Solid Edge part; units mm, degrees
sketch "Sketch1" plane through (0, 0, 0) normal (0, 0, 1) x (1, 0, 0)
  line L0 (20, -15) -> (-20, -15)
  line L1 (-20, -15) -> (-20, 15)
  line L2 (-20, 15) -> (20, 15)
  line L3 (20, 15) -> (20, -15)
extrude "Protrusion1" add sketch "Sketch1" along normal blind 2
sketch "Sketch2" plane through (0, 0, 0) normal (0, 0, -1) x (1, 0, 0)
  line L0 (6.25, -11.5) -> (6.25, 11.5)
  line L1 (6.25, 11.5) -> (-6.25, 11.5)
  line L2 (-6.25, 11.5) -> (-6.25, -11.5)
  line L3 (-6.25, -11.5) -> (6.25, -11.5)
extrude "ExtrudedProtrusion_2" add sketch "Sketch2" along normal blind 6
sketch "Sketch3" plane through (-20, 0, 1) normal (-1, 0, 0) x (0, -1, 0)
  line L0 (-15, 17.5) -> (-15, 1)
  line L1 (-15, 1) -> (15, 1)
  line L2 (15, 1) -> (15, 2.5)
  arc A0 (17, 4.5) -> (15, 2.5) centre (17, 2.5) ccw
  line L3 (18.5, 4.5) -> (17, 4.5)
  line L4 (18.5, 12.5) -> (17, 12.5)
  arc A1 (15, 14.5) -> (17, 12.5) centre (17, 14.5) ccw
  line L5 (15, 14.5) -> (15, 17.5)
  line L6 (15, 17.5) -> (-15, 17.5)
  arc A2 (18.5, 12.5) -> (18.5, 4.5) centre (18.5, 8.5) cw
  arc A3 (5.625, 5.7757) -> (5.625, 11.2243) centre (0, 8.5) cw
  arc A4 (5.625, 11.2243) -> (5.625, 5.7757) centre (6, 8.5) cw
extrude "ExtrudedProtrusion_3" add sketch "Sketch3" against normal blind 4
sketch "Sketch4" plane through (0, 0, 0) normal (0, 0, -1) x (0, -1, 0)
  circle A0 centre (-13.25, 0) radius 0.75
  circle A1 centre (13.25, 0) radius 0.75
extrude "ExtrudedCutout_1" cut sketch "Sketch4" against normal blind 30
sketch "Sketch5" plane through (0, 15, 9.25) normal (0, 1, 0) x (-1, 0, 0)
  line L0 (16, 6.25) -> (2.5, -7.25)
  line L1 (2.5, -7.25) -> (16, -7.25)
  line L2 (16, -7.25) -> (16, 6.25)
extrude "ExtrudedProtrusion_4" add sketch "Sketch5" against normal blind 3
sketch "Sketch6" plane through (0, 0, 0) normal (0, 0, -1) x (0, 1, 0)
  line L0 (-15, 20) -> (15, 20)
  line L1 (15, 20) -> (15, 6.25)
  line L2 (15, 6.25) -> (-15, 6.25)
  line L3 (-15, 6.25) -> (-15, 20)
extrude "ExtrudedCutout_2" cut sketch "Sketch6" against normal blind 11
fillet "Round_1" radius 2 2 edges at (6.25, -15, 1) (6.25, 15, 1)
fillet "Round_2" radius 2 2 edges at (-18, 15, 18.5) (-18, -15, 18.5)
sketch "Sketch7" plane through (-20, 0, 1) normal (-1, 0, 0) x (0, -1, 0)
  circle A0 centre (-8.5, 8.5) radius 1.25
  circle A1 centre (19, 8.5) radius 1.25
extrude "ExtrudedCutout_3" cut sketch "Sketch7" against normal blind 8
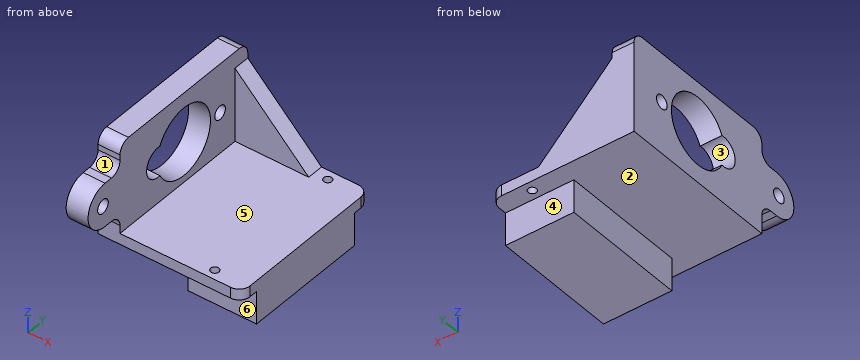
Work out the finished part from the listing and answer in its coordinate system (mm). Face numbers are marked on the shaded views. A direction names the side the tool comes from. Coordinates: 2 decimals unless noted, no trailing zeros. Loops run counter-clockwise (first coordinate to the right, second up) from the corner with the lowest first, then second, coordinate; pieces in that order, holes last. Notation, with made-up numbers: (4.5, 13.25) - (16.5, 13.25) arc R31 cw to (16.5, 42.25) - close; hole circle Ø11 at (89.5, -31.5). An arc over 180 degrees is marked (long way). Use a Markdown table: item, result.
Item 1: Find section C-C, the plane x = 0. Determine the outline of the cut face in (y, z), and give its area (3 significant figures).
Evaluation:
| item | result |
|---|---|
| outline | (-15, 0) - (-14, 0) - (-14, 2) - (-15, 2) - close; (-12.5, 0) - (-11.5, 0) - (-11.5, -6) - (11.5, -6) - (11.5, 0) - (12.5, 0) - (12.5, 2) - (-12.5, 2) - close; (14, 0) - (15, 0) - (15, 2) - (14, 2) - close |
| area | 192 mm2 |
Item 2: Find section D-D, the plane z = 0.5. Determine the outline of the cut face in (x, y), and give its area (3 significant figures).
Evaluation:
| item | result |
|---|---|
| outline | (-20, -15) - (4.25, -15) arc R2 ccw to (6.25, -13) - (6.25, 13) arc R2 ccw to (4.25, 15) - (-20, 15) - close; hole circle Ø1.5 at (0, -13.25); hole circle Ø1.5 at (0, 13.25) |
| area | 782 mm2 |
Item 3: Find section B-B, the plane y = 8.5. Determine the outline of the cut face in (x, z), and give its area (4 significant figures).
Evaluation:
| item | result |
|---|---|
| outline | (-20, 0) - (-6.25, 0) - (-6.25, -6) - (6.25, -6) - (6.25, 2) - (-16, 2) - (-16, 8.25) - (-20, 8.25) - close; (-20, 10.75) - (-16, 10.75) - (-16, 18.5) - (-20, 18.5) - close |
| area | 183.5 mm2 |
Item 4: The mould has two halves that part along Y. Classify the marked faces 1, 2 and 3: +Y half, -Y half, draft (parallel to the pull), parting line (faces both ways), or undercut.
Evaluation:
| item | result |
|---|---|
| face 1 | -Y half |
| face 2 | draft |
| face 3 | undercut |
Item 5: Given pin 1 Ø4 at (y, z) = (-19, 9.5) entering from -X; pin 2 Ø11 at (y, z) = (0, 9.5) entering from -X; pin 3 Ø7 at (x, z) = (-10.5, 6.5) entering from -Y; pin 4 Ø8 at (y, z) = (-3, 11.5) entering from +X, each flat-ended and moving along its own axis, determine where each tip first touches the part or whether it passes through.
Evaluation:
| item | result |
|---|---|
| pin 1 | stops at x = -20 |
| pin 2 | passes through |
| pin 3 | stops at y = 12 |
| pin 4 | stops at x = -16 |
Item 6: Consider probe 1 along Z at (x, y) = (-17.5, 0); probe 2 along Z at (x, y) = (-18.1, 8.5); probe 3 along X at (y, z) = (8, 6.5). Determine where each line is inside the solid, lowest interval first. Write a range as from..to.
Evaluation:
| item | result |
|---|---|
| probe 1 | z = 0..3.25, 15.75..18.5 |
| probe 2 | z = 0..8.25, 10.75..18.5 |
| probe 3 | x = -20..-16 |
Item 7: Find section A-A, the plane z = 9.5. Determine the outline of the cut face in (x, y), and give its area (3 significant figures).
Evaluation:
| item | result |
|---|---|
| outline | (-20, -22.5) - (-16, -22.5) - (-16, -20.25) - (-20, -20.25) - close; (-20, -17.75) - (-16, -17.75) - (-16, -8.75) - (-20, -8.75) - close; (-20, 6.25) - (-16, 6.25) - (-16, 7.25) - (-20, 7.25) - close; (-20, 9.75) - (-16, 9.75) - (-16, 12) - (-10, 12) - (-10, 15) - (-20, 15) - close |
| area | 88.0 mm2 |
Item 8: For the marked faces 4, 5 and 6, determine the directions among +Z, -Z, +X, -X, +Y, -Y from which every point of the face is accessible in a straight line to the end or side of a thin tool.
Evaluation:
| item | result |
|---|---|
| face 4 | -Z, +X, -X, +Y |
| face 5 | +Z, +X, -Y |
| face 6 | -Z, +X, -X, -Y |
